from build123d import *

# Parameters (mm, degrees)
SKETCH2_W                     = 76.2
SKETCH2_H                     = 76.2
BOSS_EXTRUDE1_DEPTH           = 20
CUT_EXTRUDE1_DEPTH            = 10
SKETCH4_R                     = 10
CUT_EXTRUDE2_DEPTH            = 5
TAP_DRILL_FOR_M3X0_5_TAP1_D   = 2.5
FILLET1_R                     = 5
TAP_DRILL_FOR_M3_5X0_6_TAP1_D = 2.9


with BuildPart() as part:
    # Sketch2 → Boss-Extrude1 (new body)
    with BuildSketch(Plane(origin=(0, 0, 0), x_dir=(1, 0, 0), z_dir=(0, 1, 0))):
        Rectangle(SKETCH2_W, SKETCH2_H)
    extrude(amount=BOSS_EXTRUDE1_DEPTH)

    # Sketch3 → Cut-Extrude1 (cut)
    with BuildSketch(Plane(origin=(0, 20, 0), x_dir=(1, 0, 0), z_dir=(0, 1, 0))):
        with BuildLine():
            Line((-10, -16.507271125), (10, -16.507271125))
            ThreePointArc((10, -16.507271125), (0, 19.3), (-10, -16.507271125))
        make_face()
    extrude(amount=-CUT_EXTRUDE1_DEPTH, mode=Mode.SUBTRACT)

    # Sketch4 → Cut-Extrude2 (cut)
    with BuildSketch(Plane.XZ):
        Circle(SKETCH4_R)
    extrude(amount=-CUT_EXTRUDE2_DEPTH, mode=Mode.SUBTRACT)

    # Tap Drill for M3x0.5 Tap1 (through all)
    with Locations(Plane(origin=(0, 5, 0), x_dir=(-1, 0, 0), z_dir=(0, -1, 0))):
        with Locations((0, 0)):
            Hole(TAP_DRILL_FOR_M3X0_5_TAP1_D / 2)

    # Fillet1
    fillet1_edges = [part.edges().sort_by_distance(p)[0] for p in [
        (38.1, 10, 38.1),
        (-38.1, 10, 38.1),
        (-38.1, 10, -38.1),
        (38.1, 10, -38.1),
    ]]
    fillet(fillet1_edges, radius=FILLET1_R)

    # Tap Drill for M3.5x0.6 Tap1 (through all)
    with Locations(Plane(origin=(0, 0, 0), x_dir=(-1, 0, 0), z_dir=(0, -1, 0))):
        with Locations((25, 25), (-25, -25), (-25, 25), (25, -25)):
            Hole(TAP_DRILL_FOR_M3_5X0_6_TAP1_D / 2)


solid = part.part
Geometry check sheet. Reference: the model listing, model coordinates, mm. A direction names the side the tool comes from. Round coordinates to 2 decimals unless told otherwise and drop trailing zeros. Loops run counter-clockwise (first coordinate to the right, second up) from the corner with the lowest first, then second, coordinate; pieces in that order, holes last. Notation, with made-up numbers: (-27.5, 72.5) - (-12.5, 72.5) arc R31 ccw to (-12.5, 103.5) - close; hole circle Ø2 at (-35.5, 30). An arc over 180 degrees is marked (long way). One line per question, with ' | ' between items. Start each with the question number.
1. Cross-section at C-C on z = 0. Record the cut outline in (x, y).
2. Cross-section at D-D on y = 3.5. Record the cut outline in (x, z), then the cut area to 3 significant figures.
3. Tool access check on faces 1 (the face through (-38.1, 10, 0)), 2 (the face through (2, 5, 0)), 3 (the face through (0.702, 15.07, -19.287)). Record the directions out of +Z, -Z, +X, -X, +Y, -Y that give a thin tool (end or side, any length) a straight path to the whole face; none if there is none.
4. Scan lines: line 1 (X direction, y = 4.5, z = 25); line 2 (X direction, y = 15.75, z = 0). Record each from-to range of solid material in increasing order. Write a range as [from, to].
5. Depth check by flat-ended pin: pin 1 (2.5 mm diameter, centred on x = 25, z = -25, fed in from +Y); pin 2 (3 mm diameter, centred on x = 0, z = 0, fed in from +Y); pin 3 (5 mm diameter, centred on x = -3, z = -3, fed in from -Y). Enter the tip coordinate at first touch or a pass-through.
6. Cross-section at A-A on z = -25. Record the cut outline in (x, y), then the cut area to 3 significant figures.
7. Cross-section at B-B on x = 25. Record the cut outline in (y, z), then the cut area to 3 significant figures.
8. Draft check along Z on faces 4 (the face through (-9, 20, -17.5)), 5 (the face through (0, 10, 38.1)), 6 (the face through (-2.17, 2.46, -9.76)). Enter one of: released by +Z, released by -Z, zero draft, split by the parting line, or undercut.
Taken from the geometry:
1) outline: (-38.1, 0) - (-10, 0) - (-10, 5) - (-1.25, 5) - (-1.25, 10) - (-19.3, 10) - (-19.3, 20) - (-38.1, 20) - close; (1.25, 5) - (10, 5) - (10, 0) - (38.1, 0) - (38.1, 20) - (19.3, 20) - (19.3, 10) - (1.25, 10) - close
2) outline: (-38.1, -33.1) arc R5 ccw to (-33.1, -38.1) - (33.1, -38.1) arc R5 ccw to (38.1, -33.1) - (38.1, 33.1) arc R5 ccw to (33.1, 38.1) - (-33.1, 38.1) arc R5 ccw to (-38.1, 33.1) - close; hole circle Ø2.9 at (-25, -25); hole circle Ø2.9 at (-25, 25); hole circle Ø20 at (0, 0); hole circle Ø2.9 at (25, -25); hole circle Ø2.9 at (25, 25) | area: 5,440 mm²
3) face 1: +Z, -Z, -X, +Y, -Y | face 2: -Y | face 3: +Y
4) line 1: [-38.1, -26.45], [-23.55, 23.55], [26.45, 38.1] | line 2: [-38.1, -19.3], [19.3, 38.1]
5) pin 1: through | pin 2: y = 10 | pin 3: y = 5
6) outline: (-38.1, 0) - (-26.45, 0) - (-26.45, 20) - (-38.1, 20) - close; (-23.55, 0) - (23.55, 0) - (23.55, 20) - (-23.55, 20) - close; (26.45, 0) - (38.1, 0) - (38.1, 20) - (26.45, 20) - close | area: 1,410 mm²
7) outline: (0, -38.1) - (20, -38.1) - (20, -26.45) - (0, -26.45) - close; (0, -23.55) - (20, -23.55) - (20, 23.55) - (0, 23.55) - close; (0, 26.45) - (20, 26.45) - (20, 38.1) - (0, 38.1) - close | area: 1,410 mm²
8) face 4: zero draft | face 5: released by +Z | face 6: undercut
